```python
from build123d import *

# Parameters (mm, degrees)
SKETCH1_R           = 7.5
BOSS_EXTRUDE1_DEPTH = 5
SKETCH2_R           = 3.25
CUT_EXTRUDE1_DEPTH  = 1.5
SKETCH4_R           = 8.5
BOSS_EXTRUDE2_DEPTH = 1
SKETCH3_R           = 1.6
CUT_EXTRUDE2_DEPTH  = 14.019216566


with BuildPart() as part:
    # Sketch1 → Boss-Extrude1 (new body)
    with BuildSketch(Plane(origin=(0, 0, 0), x_dir=(1, 0, 0), z_dir=(0, 1, 0))):
        with Locations(Location((0, 0, 0), (0, 0, 270))):
            Circle(SKETCH1_R)
    extrude(amount=BOSS_EXTRUDE1_DEPTH)

    # Sketch2 → Cut-Extrude1 (cut)
    with BuildSketch(Plane(origin=(0, 5, 0), x_dir=(1, 0, 0), z_dir=(0, 1, 0))):
        with Locations(Location((0, 4, 0), (0, 0, 270))):
            Circle(SKETCH2_R)
        with Locations(Location((0, -4, 0), (0, 0, 270))):
            Circle(SKETCH2_R)
    extrude(amount=-CUT_EXTRUDE1_DEPTH, mode=Mode.SUBTRACT)

    # Sketch4 → Boss-Extrude2 (add)
    with BuildSketch(Plane.XZ):
        with Locations(Location((0, 0, 0), (0, 0, 270))):
            Circle(SKETCH4_R)
    extrude(amount=-BOSS_EXTRUDE2_DEPTH)

    # Sketch3 → Cut-Extrude2 (cut, through all)
    with BuildSketch(Plane(origin=(0, 5, 0), x_dir=(1, 0, 0), z_dir=(0, 1, 0))):
        with Locations(Location((0, 4, 0), (0, 0, 270))):
            Circle(SKETCH3_R)
        with Locations(Location((0, -4, 0), (0, 0, 270))):
            Circle(SKETCH3_R)
    extrude(amount=-CUT_EXTRUDE2_DEPTH, mode=Mode.SUBTRACT)


solid = part.part
```
Design review of the part built by this model. Coordinates are the model's own, in mm. A direction names the side the tool comes from. Coordinates: 2 decimals unless noted, no trailing zeros. Order: outer loops, then holes, each group sorted by start corner. A loop starts at its lowest first (then second) coordinate and runs counter-clockwise, first axis right, second up. Notation, with made-up numbers: (-38, -27) - (0, -27) arc R24 ccw to (0, 8) - close; hole circle Ø6 at (81.25, 70). An arc over 180 degrees is marked (long way). Answer in a Markdown table with one row per item.
(1) Consider section A-A on x = 0. State the section outline as (y, z) points.
Checked values:
| item | result |
|---|---|
| outline | (0, -8.5) - (1, -8.5) - (1, -7.5) - (5, -7.5) - (5, -7.25) - (3.5, -7.25) - (3.5, -5.6) - (0, -5.6) - close; (0, -2.4) - (3.5, -2.4) - (3.5, -0.75) - (5, -0.75) - (5, 0.75) - (3.5, 0.75) - (3.5, 2.4) - (0, 2.4) - close; (0, 5.6) - (3.5, 5.6) - (3.5, 7.25) - (5, 7.25) - (5, 7.5) - (1, 7.5) - (1, 8.5) - (0, 8.5) - close |
(2) For faces 1 (the cylindrical face through (-0.61, 1.77, 5.48)), 2 (the flat face through (-1.4, 3.5, -2.6)), list the 3-axis set-ups (+Z, -Z, +X, -X, +Y, -Y) from which the entire face can be reached by the end or side of a thin tool; tool diameter is ignored.
Checked values:
| item | result |
|---|---|
| face 1 | +Y, -Y |
| face 2 | +Y |
(3) Consider section C-C on z = 0. State the section outline as (x, y) points.
Checked values:
| item | result |
|---|---|
| outline | (-8.5, 0) - (8.5, 0) - (8.5, 1) - (7.5, 1) - (7.5, 5) - (-7.5, 5) - (-7.5, 1) - (-8.5, 1) - close |
(4) Consider section B-B on z = 3.5. State the section outline as (x, y) points, plus the area to 3 significant figures.
Checked values:
| item | result |
|---|---|
| outline | (-7.75, 0) - (-1.52, 0) - (-1.52, 3.5) - (-3.21, 3.5) - (-3.21, 5) - (-6.63, 5) - (-6.63, 1) - (-7.75, 1) - close; (1.52, 0) - (7.75, 0) - (7.75, 1) - (6.63, 1) - (6.63, 5) - (3.21, 5) - (3.21, 3.5) - (1.52, 3.5) - close |
| area | 48.3 mm^2 |
(5) The part is to be moulded in two halves that separate along Z. For faces 3 (the cylindrical face through (8.428, 0.493, 1.107)), 4 (the flat face through (0, 5, 0)), 5 (the cylindrical face through (0.98, 4.26, -0.9)), say which applies: released by +Z, released by -Z, zero draft, split by the parting line, or undercut.
Checked values:
| item | result |
|---|---|
| face 3 | split by the parting line |
| face 4 | zero draft |
| face 5 | undercut |
(6) Clearance check with flat-ended pins moving along their axes: pin 1 (1 mm diameter, centred on y = 4, z = -0.5, fed in from -X); pin 2 (2 mm diameter, centred on x = -1, z = -4, fed in from +Y); pin 3 (3 mm diameter, centred on x = 0, z = 4, fed in from +Y). State where each tip first meets the part, or that it passes through.
Checked values:
| item | result |
|---|---|
| pin 1 | x = -7.5 |
| pin 2 | y = 3.5 |
| pin 3 | through |
(7) Wall thickness on line 1 along X through (y, z) = (0.8, -4); line 2 along Y through (x, z) = (-2.25, 5.5); line 3 along X through (y, z) = (4.4, 1.75): over which ranges is each line inside the solid? List them lowest first. Write a range as from..to.
Checked values:
| item | result |
|---|---|
| line 1 | -7.5..-1.6, 1.6..7.5 |
| line 2 | 0..3.5 |
| line 3 | -7.29..-2.35, 2.35..7.29 |
(8) Consider section D-D on y = 4.1. State the section outline as (x, z) points.
Checked values:
| item | result |
|---|---|
| outline | circle Ø15 at (0, 0); hole circle Ø6.5 at (0, -4); hole circle Ø6.5 at (0, 4) |
